Input: part model. Units: mm. Frame: model coordinates. Face numbers are marked on the shaded views. A direction names the side the tool comes from. Give positions to 0.01 mm unless a question says otherwise; leave off trailing zeros. Loops run counter-clockwise (first coordinate to the right, second up) from the corner with the lowest first, then second, coordinate; pieces in that order, holes last. Notation, with made-up numbers: (55, -9.75) -> (94, -9.75) arc R11 cw to (94, -2.75) -> close; hole circle Ø9 at (64, 18.5). An arc over 180 degrees is marked (long way). Answer as a JSON object with one key per item and string values. Group by question number.
```python
from build123d import *

# Parameters (mm, degrees)
PAD_DEPTH = 1
FILLET_R  = 0.8


with BuildPart() as part:
    # Sketch → Pad (new body)
    with BuildSketch(Plane.XY):
        with BuildLine():
            ThreePointArc((5.114745, -6.151372), (0, 8), (-5.114745, -6.151372))
            Line((-5.114745, -6.151372), (-3.75, -1.391941))
            ThreePointArc((-3.804226, 1.236068), (-3.999149, -0.082518), (-3.75, -1.391941))
            Line((-5.706339, 1.854102), (-3.804226, 1.236068))
            ThreePointArc((-1.854249, 5.706291), (-4.242695, 4.242586), (-5.706339, 1.854102))
            Line((-1.854249, 5.706291), (-1.236068, 3.804226))
            ThreePointArc((1.236068, 3.804226), (0, 4), (-1.236068, 3.804226))
            Line((1.853955, 5.706387), (1.236068, 3.804226))
            ThreePointArc((5.706339, 1.854102), (4.242586, 4.242695), (1.853955, 5.706387))
            Line((3.804226, 1.236068), (5.706339, 1.854102))
            ThreePointArc((3.75, -1.391941), (3.999149, -0.082518), (3.804226, 1.236068))
            Line((5.114745, -6.151372), (3.75, -1.391941))
        make_face()
    extrude(amount=PAD_DEPTH)

    # Fillet
    fillet_edges = [part.edges().sort_by_distance(p)[0] for p in [
        (-5.114745, -6.151372, 0.5),
        (-3.75, -1.391941, 0.5),
        (-3.804226, 1.236068, 0.5),
        (-5.706339, 1.854102, 0.5),
        (-1.854249, 5.706291, 0.5),
        (-1.236068, 3.804226, 0.5),
        (1.236068, 3.804226, 0.5),
        (1.853955, 5.706387, 0.5),
        (5.706339, 1.854102, 0.5),
        (3.804226, 1.236068, 0.5),
        (3.75, -1.391941, 0.5),
        (5.114745, -6.151372, 0.5),
    ]]
    fillet(fillet_edges, radius=FILLET_R)


solid = part.part
```
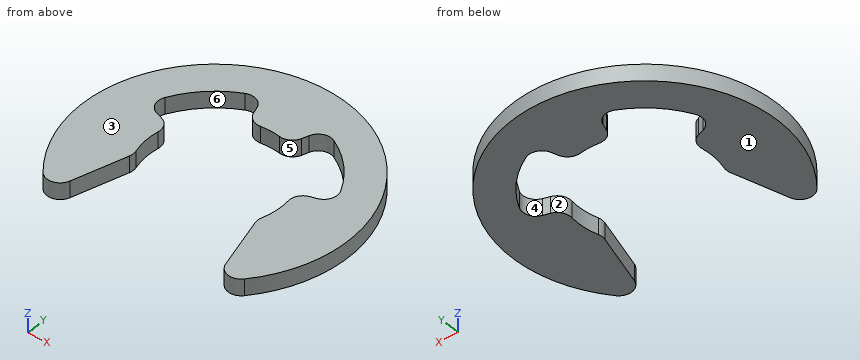
Q1. Section A-A on y = 0. Return the cut outline in (x, z).
Q2. Pull-direction query (Y, two-part tool) for the marked faces 3, 4, 5 and 6; classes: +Y half, -Y half, draft (parallel to the pull), parting line (faces both ways), or undercut.
Q3. Ray query, probe 1 along X at (y, z) = (5.25, 0.35); probe 2 along X at (y, z) = (3.5, 0.8); probe 3 along X at (y, z) = (1, 0.25). Return the intervals inside material, ascending.
Q4. Set-up query: the marked faces 1 and 2. Return all of +Z, -Z, +X, -X, +Y, -Y with unobstructed straight access to the full face (end or side cutting, diameter ignored); none if empty.
Q5. Section C-C on x = 0. Return the cut outline in (y, z), then the cut area to 3 significant figures.
Q6. Section D-D on y = -3.5. Return the cut outline in (x, z), then the cut area to 3 significant figures.
Q7. Section B-B on z = 0.5. Return the cut outline in (x, y), then the cut area to 3 significant figures.
Numbers:
{
 "1": {"outline": "(-8, 0) -> (-4, 0) -> (-4, 1) -> (-8, 1) -> close; (4, 0) -> (8, 0) -> (8, 1) -> (4, 1) -> close"},
 "2": {"face 3": "draft", "face 4": "undercut", "face 5": "-Y half", "face 6": "undercut"},
 "3": {"probe 1": "x = -6.04 to -2.9, -1.83 to 1.83, 2.9 to 6.04", "probe 2": "x = -7.19 to -4.87, 4.87 to 7.19", "probe 3": "x = -7.94 to -4.01, 4.01 to 7.94"},
 "4": {"face 1": "-Z, +X, -X, +Y, -Y", "face 2": "+Z, -Z"},
 "5": {"outline": "(4, 0) -> (8, 0) -> (8, 1) -> (4, 1) -> close", "area": "4.00 mm²"},
 "6": {"outline": "(-7.19, 0) -> (-4.35, 0) -> (-4.35, 1) -> (-7.19, 1) -> close; (4.35, 0) -> (7.19, 0) -> (7.19, 1) -> (4.35, 1) -> close", "area": "5.68 mm²"},
 "7": {"outline": "(-6.12, -5.15) arc R0.8 ccw to (-4.74, -4.85) -> (-3.82, -1.63) arc R0.8 ccw to (-3.82, -1.18) arc R4 cw to (-3.96, 0.58) arc R0.8 ccw to (-4.5, 1.46) -> (-4.89, 1.59) arc R0.8 cw to (-5.35, 2.71) arc R6 cw to (-2.71, 5.35) arc R0.8 cw to (-1.59, 4.89) -> (-1.46, 4.5) arc R0.8 ccw to (-0.58, 3.96) arc R4 cw to (0.58, 3.96) arc R0.8 ccw to (1.46, 4.5) -> (1.59, 4.89) arc R0.8 cw to (2.71, 5.35) arc R6 cw to (5.35, 2.71) arc R0.8 cw to (4.89, 1.59) -> (4.5, 1.46) arc R0.8 ccw to (3.96, 0.58) arc R4 cw to (3.82, -1.18) arc R0.8 ccw to (3.82, -1.63) -> (4.74, -4.85) arc R0.8 ccw to (6.12, -5.15) arc R8 ccw (long way) to start", "area": "90.4 mm²"}
}
